```python
from build123d import *

# Parameters (mm, degrees)
SKETCH1_W                      = 6.35
SKETCH1_H                      = 4.7625
SKETCH1_R                      = 20.6375
SKETCH1_R_2                    = 14.2875
BOSS_EXTRUDE1_DEPTH            = 6.35
SKETCH2_W                      = 6.35
SKETCH2_H                      = 9.525
BOSS_EXTRUDE2_DEPTH            = 6.35
FILLET1_R                      = 12.7
FILLET2_R                      = 11.1125
F_6_32_TAPPED_HOLE1_D          = 2.7051
F_6_32_TAPPED_HOLE1_DEPTH      = 9.398
F_6_32_TAPPED_HOLE1_TIP        = 0.81269403
FILLET3_R                      = 25.4
FILLET4_R                      = 6.35
FILLET5_R                      = 3.175
F_6_32_TAPPED_HOLE2_AT_2_COUNT = 2
F_6_32_TAPPED_HOLE2_AT_2_PITCH = 79.375


with BuildPart() as part:
    # Sketch1 → Boss-Extrude1 (new body)
    # profile 1 of 11: a face of its own
    with BuildSketch(Plane.XY):
        with Locations((-193.675, -35.71875)):
            Rectangle(SKETCH1_W, SKETCH1_H)
    # profile 2 of 11: a face of its own
    with BuildSketch(Plane.XY):
        Polygon((190.5, -38.1), (190.5, -33.3375), (-118.579686171, -33.3375), (-190.5, -33.3375), (-190.5, -38.1), align=None)
    # profile 3 of 11: a face of its own
    with BuildSketch(Plane.XY):
        with BuildLine():
            ThreePointArc((-139.7, 55.5625), (-95.25, 11.1125), (-139.7, -33.3375))
            Line((-139.7, -33.3375), (-118.579686171, -33.3375))
            ThreePointArc((-118.579686171, -33.3375), (-90.5008099, 9.968013342), (-116.535631077, 54.53233612))
            ThreePointArc((-116.535631077, 54.53233612), (-128.106367855, 55.304831818), (-139.7, 55.5625))
        make_face()
    # profile 4 of 11: a face of its own
    with BuildSketch(Plane.XY):
        with Locations((-193.675, 57.94375)):
            Rectangle(SKETCH1_W, SKETCH1_H)
    # profile 5 of 11: a face of its own
    with BuildSketch(Plane.XY):
        with BuildLine():
            Line((-190.5, 55.5625), (-139.7, 55.5625))
            ThreePointArc((-139.7, 55.5625), (-128.106367855, 55.304831818), (-116.535631077, 54.53233612))
            ThreePointArc((-116.535631077, 54.53233612), (-59.866243781, 43.050732151), (-7.116346533, 19.371732454))
            ThreePointArc((-7.116346533, 19.371732454), (-3.614019765, 20.318594129), (0, 20.6375))
            ThreePointArc((0, 20.6375), (-67.085973021, 50.210624965), (-139.7, 60.325))
            Line((-139.7, 60.325), (-190.5, 60.325))
            Line((-190.5, 60.325), (-190.5, 55.5625))
        make_face()
    # profile 6 of 11: a face of its own
    with BuildSketch(Plane.XY):
        Circle(SKETCH1_R)
        Circle(SKETCH1_R_2, mode=Mode.SUBTRACT)
    # profile 7 of 11: a face of its own
    with BuildSketch(Plane.XY):
        with BuildLine():
            Line((-3.175, -33.3375), (3.175, -33.3375))
            Line((3.175, -33.3375), (3.175, -20.391806719))
            ThreePointArc((3.175, -20.391806719), (0, -20.6375), (-3.175, -20.391806719))
            Line((-3.175, -20.391806719), (-3.175, -33.3375))
        make_face()
    # profile 8 of 11: a face of its own
    with BuildSketch(Plane.XY):
        with BuildLine():
            ThreePointArc((116.535631077, 54.53233612), (128.106367855, 55.304831818), (139.7, 55.5625))
            Line((139.7, 55.5625), (190.5, 55.5625))
            Line((190.5, 55.5625), (190.5, 60.325))
            Line((190.5, 60.325), (139.7, 60.325))
            ThreePointArc((139.7, 60.325), (67.085973021, 50.210624965), (0, 20.6375))
            ThreePointArc((0, 20.6375), (3.614019765, 20.318594129), (7.116346533, 19.371732454))
            ThreePointArc((7.116346533, 19.371732454), (59.866243781, 43.050732151), (116.535631077, 54.53233612))
        make_face()
    # profile 9 of 11: a face of its own
    with BuildSketch(Plane.XY):
        with BuildLine():
            Line((118.579686171, -33.3375), (139.7, -33.3375))
            ThreePointArc((139.7, -33.3375), (95.25, 11.1125), (139.7, 55.5625))
            ThreePointArc((139.7, 55.5625), (128.106367855, 55.304831818), (116.535631077, 54.53233612))
            ThreePointArc((116.535631077, 54.53233612), (90.5008099, 9.968013342), (118.579686171, -33.3375))
        make_face()
    # profile 10 of 11: a face of its own
    with BuildSketch(Plane.XY):
        with Locations((193.675, 57.94375)):
            Rectangle(SKETCH1_W, SKETCH1_H)
    # profile 11 of 11: a face of its own
    with BuildSketch(Plane.XY):
        with Locations((193.675, -35.71875)):
            Rectangle(SKETCH1_W, SKETCH1_H)
    extrude(amount=-BOSS_EXTRUDE1_DEPTH)

    # Sketch2 → Boss-Extrude2 (add)
    with BuildSketch(Plane.XY):
        with Locations((-187.325, -28.575)):
            Rectangle(SKETCH2_W, SKETCH2_H)
        with Locations((-187.325, 50.8)):
            Rectangle(SKETCH2_W, SKETCH2_H)
        with Locations((187.325, 50.8)):
            Rectangle(SKETCH2_W, SKETCH2_H)
        with Locations((187.325, -28.575)):
            Rectangle(SKETCH2_W, SKETCH2_H)
    extrude(amount=-BOSS_EXTRUDE2_DEPTH)

    # Fillet1
    # the kernel refuses this fillet: 12.7 mm, written as the material it adds along each edge
    with BuildSketch(Plane(origin=(-184.15, 55.5625, 0), x_dir=(1, 0, 0), z_dir=(0, 0, -1)), Plane(origin=(184.15, -33.3375, 0), x_dir=(-1, 0, 0), z_dir=(0, 0, -1))) as fillet1_piece_1:
        with BuildLine():
            CenterArc((12.296722124, 12.7), FILLET1_R, 194.477512186, 75.522487814)
            Line((0, 9.525), (-0.245934442, 9.4615))
            ThreePointArc((-0.245934442, 9.4615), (-0.254, 4.7625), (-0.254, 0))
            Line((-0.254, 0), (0, -0.254))
            Line((0, -0.254), (12.296722124, -0.254))
            Line((12.296722124, -0.254), (12.296722124, 0))
        make_face()
    extrude(amount=6.35)
    with BuildSketch(Plane(origin=(184.15, 55.5625, 0), x_dir=(-1, 0, 0), z_dir=(0, 0, -1)), Plane(origin=(-184.15, -33.3375, 0), x_dir=(1, 0, 0), z_dir=(0, 0, -1))) as fillet1_piece_2:
        with BuildLine():
            CenterArc((12.296722124, -12.7), FILLET1_R, 90, 75.522487814)
            Line((0, -9.525), (-0.245934442, -9.4615))
            ThreePointArc((-0.245934442, -9.4615), (-0.254, -4.7625), (-0.254, 0))
            Line((-0.254, 0), (0, 0.254))
            Line((0, 0.254), (12.296722124, 0.254))
            Line((12.296722124, 0.254), (12.296722124, 0))
        make_face()
    extrude(amount=6.35)

    # Fillet2
    # the kernel refuses this fillet: 11.1125 mm, written as the material it takes off along each edge
    with BuildSketch(Plane(origin=(184.15, -23.8125, 15.875), x_dir=(-0.43306748122172567, -0.9013615016785831, 0), z_dir=(0, 0, -1)), Plane(origin=(-184.15, 46.0375, 15.875), x_dir=(0.43306748122172517, 0.9013615016785834, 0), z_dir=(0, 0, -1))) as fillet2_piece_1:
        with BuildLine():
            CenterArc((7.082527166, -10.901433526), FILLET2_R, 101.184876129, 51.043876357)
            Line((-2.749978506, -5.723645536), (-2.946628619, -5.620089776))
            ThreePointArc((-2.946628619, -5.620089776), (-1.575316847, -2.76557352), (-0.200327594, 0.096249248))
            Line((-0.200327594, 0.096249248), (0.043111035, 0.218028671))
            ThreePointArc((0.043111035, 0.218028671), (2.46348771, -0.018968828), (4.883864385, 0.218028671))
            Line((4.883864385, 0.218028671), (4.92697542, 0))
        make_face()
    extrude(amount=38.1, mode=Mode.SUBTRACT)
    with BuildSketch(Plane(origin=(184.15, 46.0375, 15.875), x_dir=(1, 0, 0), z_dir=(0, 0, -1)), Plane(origin=(-184.15, -23.8125, 15.875), x_dir=(-1, 0, 0), z_dir=(0, 0, -1))) as fillet2_piece_2:
        with BuildLine():
            CenterArc((6.758920293, -11.10497368), FILLET2_R, 92.108859198, 51.043876357)
            Line((-2.133712835, -4.440985963), (-2.311565498, -4.307706209))
            ThreePointArc((-2.311565498, -4.307706209), (-1.049758647, -2.228707764), (-0.215192637, 0.0555625))
            Line((-0.215192637, 0.0555625), (0, 0.22225))
            ThreePointArc((0, 0.22225), (3.175, 0.22225), (6.341821594, 0.222099474))
            Line((6.341821594, 0.222099474), (6.35, 0))
        make_face()
    extrude(amount=38.1, mode=Mode.SUBTRACT)

    # #6-32 Tapped Hole1
    with Locations(Plane(origin=(0, -38.1, 0), x_dir=(-1, 0, 0), z_dir=(0, -1, 0))):
        with Locations((82.55, 3.175)):
            Hole(F_6_32_TAPPED_HOLE1_D / 2, depth=F_6_32_TAPPED_HOLE1_DEPTH)
            with Locations((0, 0, -(F_6_32_TAPPED_HOLE1_DEPTH + F_6_32_TAPPED_HOLE1_TIP / 2))):  # 118° drill point
                Cone(0, F_6_32_TAPPED_HOLE1_D / 2, F_6_32_TAPPED_HOLE1_TIP, mode=Mode.SUBTRACT)

    # Fillet3
    fillet3_edges = [part.edges().sort_by_distance(p)[0] for p in [
        (0, 20.6375, -3.175),
    ]]
    fillet(fillet3_edges, radius=FILLET3_R)

    # Fillet4
    fillet4_edges = [part.edges().sort_by_distance(p)[0] for p in [
        (3.175, -20.391806719, -3.175),
        (3.175, -33.3375, -3.175),
        (7.116346533, 19.371732454, -3.175),
        (-3.175, -33.3375, -3.175),
        (-3.175, -20.391806719, -3.175),
        (-7.116346533, 19.371732454, -3.175),
    ]]
    fillet(fillet4_edges, radius=FILLET4_R)

    # Fillet5
    fillet5_edges = [part.edges().sort_by_distance(p)[0] for p in [
        (118.579686171, -33.3375, -3.175),
        (116.535631077, 54.53233612, -3.175),
        (-116.535631077, 54.53233612, -3.175),
        (-118.579686171, -33.3375, -3.175),
    ]]
    fillet(fillet5_edges, radius=FILLET5_R)

    # Sketch7 → #6-32 Tapped Hole2 (revolve, cut)
    with BuildSketch(Plane(origin=(190.5, -28.575, -3.175), x_dir=(0, 0, -1), z_dir=(0, 1, 0))):
        Polygon((0, 0), (0, 10.21069403), (1.35255, 9.398), (1.35255, 7.112), (1.7526, 7.112), (1.7526, 0), align=None)
    f_6_32_tapped_hole2 = revolve(axis=Axis((196.85, -28.575, -3.175), (-1, 0, 0)), mode=Mode.SUBTRACT)

    # #6-32 Tapped Hole2 at 2: #6-32 Tapped Hole2 ×2
    with Locations(*[(0, i * F_6_32_TAPPED_HOLE2_AT_2_PITCH, 0) for i in range(1, F_6_32_TAPPED_HOLE2_AT_2_COUNT)]):
        add(f_6_32_tapped_hole2, mode=Mode.SUBTRACT)

    # Mirror1: #6-32 Tapped Hole2 across plane
    add(f_6_32_tapped_hole2.mirror(Plane(origin=(0, 0, 0), x_dir=(0, 0, 1), z_dir=(1, 0, 0))), mode=Mode.SUBTRACT)

    # Mirror1 copy 1 sketch → Mirror1 copy 1 (revolve, cut)
    with BuildSketch(Plane(origin=(-190.5, 50.8, -3.175), x_dir=(0, 0, -1), z_dir=(0, 1, 0))):
        Polygon((0, 0), (0, -10.21069403), (1.35255, -9.398), (1.35255, -7.112), (1.7526, -7.112), (1.7526, 0), align=None)
    revolve(axis=Axis((-196.85, 50.8, -3.175), (-1, 0, 0)), mode=Mode.SUBTRACT)


solid = part.part
```
Part model, mm, in its own coordinate system. A direction names the side the tool comes from. Round coordinates to 2 decimals unless told otherwise and drop trailing zeros. Order: outer loops, then holes, each group sorted by start corner. A loop starts at its lowest first (then second) coordinate and runs counter-clockwise, first axis right, second up. Notation, with made-up numbers: M 13.5,63 L 51.5,63 A25 cw 51.5,97 Z; hole C -25,-17.5 d6. An arc over 180 degrees is marked long. Put each result on its own line as item: value. Start each with the question number.
1. Slice it at B-B on y = 0. List the corners of the cut face in (x, z).
2. Tool access for faces 1 (the face through (-156, -33.338, -3)), 2 (the face through (-190.5, -30, -5)), 3 (the face through (194, -33.338, -3)): list every direction of +Z, -Z, +X, -X, +Y, -Y with a clear straight run to the whole face (end or side of a thin tool).
3. Two-plate mould, pull along Y, no slides. Class faces 4 (the face through (190.5, 50, -5)), 5 (the face through (-168, 60.325, -3)), 6 (the face through (-20.215, -4.156, -3.131)): +Y half, -Y half, draft (parallel to the pull), parting line (faces both ways), or undercut.
4. Slice it at D-D on x = 76. List the corners of the cut face in (y, z), then the cut area to 3 significant figures.
5. Slice it at C-C on y = 36.5. List the corners of the cut face in (x, z), then the cut area to 3 significant figures.
6. Drop flat-ended pins along their axis: pin 1 (3 mm diameter, centred on y = 30, z = -2.5, fed in from -X); pin 2 (3 mm diameter, centred on y = -28.575, z = -3.175, fed in from -X); pin 3 (1.9 mm diameter, centred on y = -26, z = -4.5, fed in from -X). Give the stop position or say it passes through.
7. Drill centre lines: probe 1 along Y at (x, z) = (156.5, -2.25) (1 decimal); probe 2 along Z at (x, y) = (-185.75, 50.8); probe 3 along X at (y, z) = (-4, -3.5). Where is each one in solid material? Low to high. Write a range as [from, to].
8. Slice it at A-A on x = 136. List the corners of the cut face in (y, z).
Findings:
1. outline: M -96.66,-6.35 L -91.76,-6.35 L -91.76,0 L -96.66,0 Z; M -20.64,-6.35 L -14.29,-6.35 L -14.29,0 L -20.64,0 Z; M 14.29,-6.35 L 20.64,-6.35 L 20.64,0 L 14.29,0 Z; M 91.76,-6.35 L 96.66,-6.35 L 96.66,0 L 91.76,0 Z
2. face 1: +Z, -Z
2. face 2: +Z, -Z, -X
2. face 3: +Z, -Z, +X
3. face 4: undercut
3. face 5: +Y half
3. face 6: undercut
4. outline: M -38.1,-6.35 L -33.34,-6.35 L -33.34,0 L -38.1,0 Z; M 47.67,-6.35 L 52.58,-6.35 L 52.58,0 L 47.67,0 Z
4. area: 61.4 mm2
5. outline: M -103.21,-6.35 L -97.54,-6.35 L -97.54,0 L -103.21,0 Z; M -41.79,-6.35 L -29.73,-6.35 L -29.73,0 L -41.79,0 Z; M 29.73,-6.35 L 41.79,-6.35 L 41.79,0 L 29.73,0 Z; M 97.54,-6.35 L 103.21,-6.35 L 103.21,0 L 97.54,0 Z
5. area: 225 mm2
6. pin 1: x = -100.2
6. pin 2: x = -183.39
6. pin 3: x = -190.5
7. probe 1: [-38.1, -33.3], [55.6, 60.3]
7. probe 2: [-6.35, -4.93], [-1.42, 0]
7. probe 3: [-97.9, -92.87], [-20.25, -13.72], [13.72, 20.25], [92.87, 97.9]
8. outline: M -38.1,-6.35 L -33.18,-6.35 L -33.18,0 L -38.1,0 Z; M 55.41,-6.35 L 60.3,-6.35 L 60.3,0 L 55.41,0 Z
